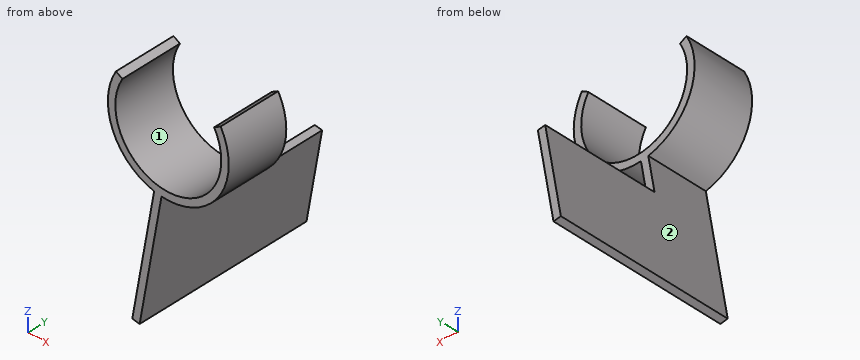
Autodesk Fusion 360 part; units mm, degrees
sketch "Ring" plane through (0, 0, 0) normal (0, 1, 0) x (1, 0, 0)
  circle A0 centre (0, 0) radius 17.05
  circle A1 centre (0, 0) radius 19.45
  dimension "d234" = 34.1
  dimension "d235" = 38.9
extrude "Ring (1)" add sketch "Ring" along normal mid plane 20
sketch "Mouth" plane through (0, 0, 0) normal (0, 1, 0) x (1, 0, 0)
  line L0 (0, 0) -> (42.3486, -24.45)
  line L1 (42.3486, -24.45) -> (0, -48.9)
  line L2 (0, -48.9) -> (-42.3486, -24.45)
  line L3 (-42.3486, -24.45) -> (0, 0)
  line L4 (0, 0) -> (0, -48.9) construction
  dimension "d238" = 48.9
  dimension "d239" = 48.9
  dimension "d240" = 48.9
  dimension "d241" = 60
  dimension "d242" = 60
extrude "Mouth (1)" cut sketch "Mouth" along normal mid plane 30
ref_plane "WorkPlane3" through (0, 12.125, 0) normal (-0.1736, 0, -0.9848) x (0, 1, 0)
sketch "Stem section" plane through (0, 0, 0) normal (-0.1736, 0, -0.9848) x (0, 1, 0)
  line L0 (1.75, 0) -> (22.5, 0) construction
  line L1 (-10, 1.2) -> (10, 1.2)
  line L2 (10, 1.2) -> (10, -1.2)
  line L3 (10, -1.2) -> (-10, -1.2)
  line L4 (-10, -1.2) -> (-10, 1.2)
  line L5 (0, 0) -> (0, 4.8) construction
  dimension "d247" = 2.4
  dimension "d248" = 4.8
  dimension "d249" = 20
extrude "Stem" add sketch "Stem section" along normal blind 12.7 from surface at 18.25
sketch "Face section" plane through (0, 0, 0) normal (-0.1736, 0, -0.9848) x (0, 1, 0)
  line L0 (1.75, 0) -> (22.5, 0) construction
  line L1 (-10, 1.2) -> (48, 1.2)
  line L2 (48, 1.2) -> (48, -1.2)
  line L3 (48, -1.2) -> (-10, -1.2)
  line L4 (-10, -1.2) -> (-10, 1.2)
  line L5 (-10, -1.2) -> (-10, 1.2) construction
  dimension "d253" = 2.4
  dimension "d254" = 58
extrude "Label face" add sketch "Face section" along normal blind 29 from surface at 30.95
equation "clipWidth = 20.0 mm"
equation "faceWidth = 58.0 mm"
equation "rodOuterDiameter = 33.4 mm"
equation "clipClearance = 0.7 mm"
equation "clipWall = 2.4 mm"
equation "mouthHalfAngleDeg = 60.0 deg"
equation "paddleThickness = 2.4 mm"
equation "stemEndRadius = ( rodOuterDiameter + clipClearance + 2 * clipWall ) / 2 + stemLength"
equation "faceEndRadius = stemEndRadius + faceHeight"
equation "paddleAngleDeg = 100.0 deg"
equation "stemStartRadius = ( rodOuterDiameter + clipClearance ) / 2 + clipWall / 2"
equation "stemLength = 11.5 mm"
equation "faceHeight = 29.0 mm"
equation "d234 = rodOuterDiameter + clipClearance"
equation "d235 = rodOuterDiameter + clipClearance + 2 * clipWall"
equation "d236 = clipWidth"
equation "d238 = Linear Dimension-2"
equation "d239 = Linear Dimension-3"
equation "d240 = Linear Dimension-4"
equation "d241 = mouthHalfAngleDeg"
equation "d242 = mouthHalfAngleDeg"
equation "d243 = clipWidth + 10 mm"
equation "d245 = paddleAngleDeg"
equation "d247 = paddleThickness"
equation "d248 = paddleThickness * 2"
equation "d249 = clipWidth"
equation "d250 = stemStartRadius"
equation "d251 = stemEndRadius - stemStartRadius"
equation "d253 = paddleThickness"
equation "d254 = faceWidth"
equation "d255 = stemEndRadius"
equation "d256 = faceEndRadius - stemEndRadius"
Verification items for the finished model (mm, model axes). Face numbers are marked on the shaded views. Give positions to 0.01 mm unless a question says otherwise; leave off trailing zeros. Order: outer loops, then holes, each group sorted by start corner. A loop starts at its lowest first (then second) coordinate and runs counter-clockwise, first axis right, second up. Notation, with made-up numbers: (-39, -3.5) -> (0, -3.5) arc R27 cw to (0, 24.5) -> close; hole circle Ø9 at (37, 43). An arc over 180 degrees is marked (long way). Use a Markdown table: item, result.
1) Section check B-B, the plane y = 3.5. Record the boundary of the cut face in (x, z) (3 decimals), then the cut area to 3 significant figures.
Results:
| item | result |
|---|---|
| outline | (-16.844, 9.725) arc R19.45 ccw to (-4.553, -18.91) -> (-11.592, -58.831) -> (-9.228, -59.248) -> (-2.189, -19.326) arc R19.45 ccw to (16.844, 9.725) -> (14.766, 8.525) arc R17.05 cw (long way) to (-14.766, 8.525) -> close |
| area | 281 mm² |
2) Material ranges on probe 1 along X at (y, z) = (-0.5, 0); probe 2 along Z at (x, y) = (0, 4.5); probe 3 along X at (y, z) = (6.5, -7), recorded low to high.
Results:
| item | result |
|---|---|
| probe 1 | -19.45 to -17.05, 17.05 to 19.45 |
| probe 2 | -19.45 to -17.05 |
| probe 3 | -18.15 to -15.55, 15.55 to 18.15 |
3) Section check C-C, the plane x = -8. Record the boundary of the cut face in (y, z).
Results:
| item | result |
|---|---|
| outline | (-10, -52.28) -> (48, -52.28) -> (48, -38.46) -> (-10, -38.46) -> close; (-10, -17.73) -> (10, -17.73) -> (10, -15.06) -> (-10, -15.06) -> close |
4) Section check D-D, the plane x = 0. Record the boundary of the cut face in (y, z), then the cut area to 3 significant figures.
Results:
| item | result |
|---|---|
| outline | (-10, -19.45) -> (10, -19.45) -> (10, -17.05) -> (-10, -17.05) -> close |
| area | 48.0 mm² |
5) Section check A-A, the plane z = 0. Record the boundary of the cut face in (x, y), then the cut area to 3 significant figures.
Results:
| item | result |
|---|---|
| outline | (-19.45, -10) -> (-17.05, -10) -> (-17.05, 10) -> (-19.45, 10) -> close; (17.05, -10) -> (19.45, -10) -> (19.45, 10) -> (17.05, 10) -> close |
| area | 96.0 mm² |
6) Depth check by flat-ended pin: pin 1 Ø12 at (x, z) = (4.5, -11) entering from +Y; pin 2 Ø1.5 at (y, z) = (11.5, -51.5) entering from -X. Enter the tip coordinate at first touch or a pass-through.
Results:
| item | result |
|---|---|
| pin 1 | y = 10 |
| pin 2 | x = -10.43 |
7) Mould release check, pull along X, two halves, no side actions. Record for the marked faces 1 and 2: pulls with the +X half, pulls with the -X half, needs draft (parallel to the pull), parting line crosses it, or undercut.
Results:
| item | result |
|---|---|
| face 1 | undercut |
| face 2 | pulls with the -X half |
